Build history of the part. All positions in model axes, mm. A direction names the side the tool comes from. Give positions to 0.01 mm unless a question says otherwise; leave off trailing zeros. Write each loop counter-clockwise with the first axis right and the second up, starting at its lowest first coordinate (ties: lowest second). Pieces come first, ordered by that corner, then holes. Notation, with made-up numbers: (78.5, 22.5) -> (121.5, 22.5) arc R14 ccw to (121.5, 35.5) -> close; hole circle Ø4 at (-39, 6.5). An arc over 180 degrees is marked (long way). Write item = value, one per line. Start each with the question number.
Q1. Wall check: line 1 (Y direction, x = -220.35, z = 25); line 2 (Z direction, x = -226, y = -4.5); line 3 (X direction, y = -0.5, z = 8). Give the ranges that are in metal, low to high.
Q2. Saw through at C-C, the plane x = -229. List the corners of the cut face in (y, z), then the cut area to 3 significant figures.
Q3. Saw through at A-A, the plane y = -0.5. List the corners of the cut face in (x, z).
Q4. Drop flat-ended pins along their axis: P1, Ø5, axis at y = 3.5, z = 9, coming from the -X side; P2, Ø1, axis at x = -229.5, y = 5, coming from the +Z side; P3, Ø2, axis at y = 13.33, z = 25, coming from the +X side. Give the stop position or say it passes through.
Q5. Mould opens along Z. For faces 4 (the face through (-231, 0, 0)), 5 (the face through (-220.293, 0.055, 6.985)), 6 (the face through (-238.5, 16, 0.5)) say: pulls with the +Z half, pulls with the -Z half, needs draft (parallel to the pull), parting line crosses it, or undercut.
Q6. Tool access for faces 1 (the face through (-220.29, 14.38, 24.33)), 2 (the face through (-238.5, -16, 0.5)), 3 (the face through (-220.8, 0, 16)): list every direction of +Z, -Z, +X, -X, +Y, -Y with a clear straight run to the whole face (end or side of a thin tool).
Q7. Saw through at D-D, the plane y = 15.9. List the corners of the cut face in (x, z), then the cut area to 3 significant figures.
Q8. Saw through at B-B, the plane z = 24.75. List the corners of the cut face in (x, y), then the cut area to 3 significant figures.
from build123d import *

# Parameters (mm, degrees)
SKETCH1_W                    = 20
SKETCH1_H                    = 20.5
BASE_FLANGE1_DEPTH           = 1
EDGE_FLANGE1_STRIP_W         = 5.4732
EDGE_FLANGE1_STRIP_H         = 1
EDGE_FLANGE1_STRIP_CUT_DEPTH = 20.5
EDGE_FLANGE1_DEPTH           = 20.5
CUT_EXTRUDE1_DEPTH           = 42.003048667
CUT_EXTRUDE1_DEPTH_BACK      = 10
CUT_EXTRUDE2_DEPTH           = 1
M3_TAPPED_HOLE1_D            = 2.5


# Sheet-metal steps are written as plain solids
with BuildPart() as part:
    # Sketch1 → Base-Flange1 (new body)
    with BuildSketch(Plane.XY):
        with Locations((-229.8, 10.25)):
            Rectangle(SKETCH1_W, SKETCH1_H)
    extrude(amount=BASE_FLANGE1_DEPTH)

    # Edge-Flange1 strip (across the edge) → Edge-Flange1 strip cut (cut)
    with BuildSketch(Plane(origin=(-219.8, 0, 1), x_dir=(-1, 0, 0), z_dir=(0, 1, 0))):
        with Locations((-1, -0.5)):
            Rectangle(EDGE_FLANGE1_STRIP_W, EDGE_FLANGE1_STRIP_H)
    extrude(amount=EDGE_FLANGE1_STRIP_CUT_DEPTH, mode=Mode.SUBTRACT)

    # Edge-Flange1 section (across the edge) → Edge-Flange1 (add)
    with BuildSketch(Plane(origin=(-219.8, 0, 1), x_dir=(-1, 0, 0), z_dir=(0, 1, 0))):
        with BuildLine():
            Line((0, 0.7366), (0, 29))
            Line((0, 29), (1, 29))
            Line((1, 29), (1, 0.7366))
            ThreePointArc((1, 0.7366), (1.215745145, 0.215745145), (1.7366, 0))
            Line((1.7366, 0), (1.7366, -1))
            ThreePointArc((1.7366, -1), (0.508638364, -0.491361636), (0, 0.7366))
        make_face()
    extrude(amount=EDGE_FLANGE1_DEPTH)

    # Sketch9 → Cut-Extrude1 (cut, two sides: drawn at the far end of the back side and taken through both)
    with BuildSketch(Plane.ZY.offset(220.8).offset(-CUT_EXTRUDE1_DEPTH_BACK)):
        with BuildLine():
            Line((-80.481011606, 29.141419193), (1.7366, 20.5))
            Line((1.7366, 20.5), (22.836227706, 18.282339766))
            ThreePointArc((22.836227706, 18.282339766), (27.945158604, 15.679209453), (30, 10.326164603))
            Line((30, 10.326164603), (30, 0))
            Line((30, 0), (30, -82.670489196))
            Line((30, -82.670489196), (147.611596884, 33.541177232))
            Line((147.611596884, 33.541177232), (37.130585278, 145.353085621))
            Line((37.130585278, 145.353085621), (-80.481011606, 29.141419193))
        make_face()
    extrude(amount=CUT_EXTRUDE1_DEPTH + CUT_EXTRUDE1_DEPTH_BACK, mode=Mode.SUBTRACT)

    # Sketch11 → Cut-Extrude2 (cut)
    with BuildSketch(Plane.XY.offset(1)):
        with BuildLine():
            Line((-229.5, 18.9), (-235.5, 18.9))
            ThreePointArc((-235.5, 18.9), (-238.5, 15.9), (-235.5, 12.9))
            Line((-235.5, 12.9), (-229.5, 12.9))
            ThreePointArc((-229.5, 12.9), (-226.5, 15.9), (-229.5, 18.9))
        make_face()
    extrude(amount=-CUT_EXTRUDE2_DEPTH, mode=Mode.SUBTRACT)

    # Mirror1: part across plane


with BuildPart() as part_1:
    add(part.part)
    add(part.part.mirror(Plane(origin=(-239.8, 0, 1), x_dir=(0, 0, 1), z_dir=(0, 1, 0))))

    # M3 Tapped Hole1 (through all)
    with Locations(Plane.ZY.offset(220.8)):
        with Locations((5.7366, 0), (25, 13.326164603), (25, -13.326164603)):
            Hole(M3_TAPPED_HOLE1_D / 2)


solid = part_1.part
Report:
q1.line_1 = -17.74 to -14.58, -12.08 to 12.08, 14.58 to 17.74
q1.line_2 = 0 to 1
q1.line_3 = -220.8 to -219.8
q2.outline = (-20.5, 0) -> (-18.86, 0) -> (-18.86, 1) -> (-20.5, 1) -> close; (-12.94, 0) -> (12.94, 0) -> (12.94, 1) -> (-12.94, 1) -> close; (18.86, 0) -> (20.5, 0) -> (20.5, 1) -> (18.86, 1) -> close
q2.area = 29.2 mm2
q3.outline = (-239.8, 0) -> (-221.54, 0) arc R1.74 ccw to (-219.8, 1.74) -> (-219.8, 4.59) -> (-220.8, 4.59) -> (-220.8, 1.74) arc R0.74 cw to (-221.54, 1) -> (-239.8, 1) -> close; (-220.8, 6.88) -> (-219.8, 6.88) -> (-219.8, 30) -> (-220.8, 30) -> close
q4.P1 = -220.8
q4.P2 = 1
q4.P3 = through
q5.face_4 = pulls with the -Z half
q5.face_5 = undercut
q5.face_6 = needs draft
q6.face_1 = +X, -X
q6.face_2 = +Z, -Z
q6.face_3 = +Z, -X, +Y, -Y
q7.outline = (-239.8, 0) -> (-238.5, 0) -> (-238.5, 1) -> (-239.8, 1) -> close; (-226.5, 0) -> (-221.54, 0) arc R1.74 ccw to (-219.8, 1.74) -> (-219.8, 27.74) -> (-220.8, 27.74) -> (-220.8, 1.74) arc R0.74 cw to (-221.54, 1) -> (-226.5, 1) -> close
q7.area = 34.2 mm2
q8.outline = (-220.8, -17.84) -> (-219.8, -17.84) -> (-219.8, -14.55) -> (-220.8, -14.55) -> close; (-220.8, -12.1) -> (-219.8, -12.1) -> (-219.8, 12.1) -> (-220.8, 12.1) -> close; (-220.8, 14.55) -> (-219.8, 14.55) -> (-219.8, 17.84) -> (-220.8, 17.84) -> close
q8.area = 30.8 mm2
